```python
from build123d import *

# Parameters (mm, degrees)
F1_DEPTH = 190.5
F2_DEPTH = 127
F0_W     = 63.5
F0_H     = 63.5
F3_DEPTH = 101.6
F4_DEPTH = 25.4
F6_DEPTH = 63.5
F0_H_2   = 31.75
F7_DEPTH = 95.25


with BuildPart() as f1:
    # F0 (on Front) → F1 (new body)
    with BuildSketch(Plane.XZ):
        Polygon((0, 63.5), (0, 0), (95.25, 0), (95.25, 31.75), (158.75, 31.75), (158.75, 0), (254, 0), (254, 31.75), (317.5, 31.75), (317.5, 63.5), (254, 63.5), (190.5, 63.5), (127, 63.5), (63.5, 63.5), align=None)
    extrude(amount=F1_DEPTH)

    # F0 (on Front) → F2 (join)
    with BuildSketch(Plane.XZ):
        Polygon((0, 190.5), (0, 63.5), (63.5, 63.5), (63.5, 127), (63.5, 190.5), align=None)
    extrude(amount=F2_DEPTH)

    # F0 (on Front) → F3 (join)
    with BuildSketch(Plane.XZ):
        with Locations((95.25, 95.25)):
            Rectangle(F0_W, F0_H)
        with Locations((222.25, 95.25)):
            Rectangle(F0_W, F0_H)
    extrude(amount=F3_DEPTH)

    # F0 (on Front) → F4 (join)
    with BuildSketch(Plane.XZ):
        with Locations((158.75, 95.25)):
            Rectangle(F0_W, F0_H)
    extrude(amount=F4_DEPTH)

    # F5 (on face) → F6 (cut)
    with BuildSketch(Plane.XY.offset(127)):
        Polygon((254, -25.4), (190.5, -101.6), (254, -101.6), align=None)
    extrude(amount=-F6_DEPTH, mode=Mode.SUBTRACT)

    # F0 (on Front) → F7 (join)
    with BuildSketch(Plane.XZ):
        with Locations((285.75, 15.875)):
            Rectangle(F0_W, F0_H_2)
    extrude(amount=F7_DEPTH)


solid = f1.part
```
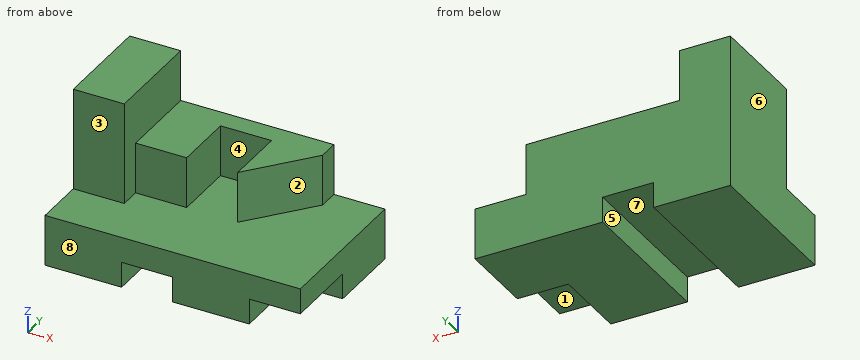
Geometry: final body of the model. Coordinates: model frame, mm. Face numbers are marked on the shaded views. A direction names the side the tool comes from. Round coordinates to 2 decimals unless told otherwise and drop trailing zeros. Loops run counter-clockwise (first coordinate to the right, second up) from the corner with the lowest first, then second, coordinate; pieces in that order, holes last.
Item 1: Section B-B, the plane y = -133.5. Output: boundary loops of the cut face in (x, z).
Checked values:
outline: (0, 0) - (95.25, 0) - (95.25, 31.75) - (158.75, 31.75) - (158.75, 0) - (254, 0) - (254, 31.75) - (317.5, 31.75) - (317.5, 63.5) - (0, 63.5) - close
Item 2: Mould query, pull axis X, two halves, no side actions, for the marked faces 6, 7 and 8. Classes: released by +X, released by -X, zero draft, split by the parting line, or undercut.
Checked values:
face 6: released by -X
face 7: undercut
face 8: zero draft
Item 3: Line query: L1, parallel to X at y = -102, z = 26.5; L2, parallel to Z at x = 255.5, y = -149.5; L3, parallel to Z at x = 282.5, y = -15. Output: solid intervals per line, ascending.
Checked values:
L1: x = 0 to 95.25, 158.75 to 254
L2: z = 31.75 to 63.5
L3: z = 0 to 63.5
Item 4: Section A-A, the plane z = 85. Output: boundary loops of the cut face in (x, y).
Checked values:
outline: (0, -127) - (63.5, -127) - (63.5, -101.6) - (127, -101.6) - (127, -25.4) - (190.5, -25.4) - (190.5, -101.6) - (254, -25.4) - (254, 0) - (0, 0) - close
Item 5: Contact query for flat-ended pins moving along their axis: P1, Ø20.5, axis at y = -13.5, z = 84.5, coming from the +X side; P2, Ø1.5, axis at y = -106, z = 131.5, coming from the -X side; P3, Ø19, axis at x = 173.5, z = 87, coming from the -Y side; P4, Ø16, axis at x = 280, z = 18, coming from the -Y side. Output: stop coordinate, or through.
Checked values:
P1: stops at x = 254
P2: stops at x = 0
P3: stops at y = -25.4
P4: stops at y = -95.25
Item 6: Reachability of the marked faces 1, 2, 3, 4 and 5 from +Z, -Z, +X, -X, +Y, -Y: full face, straight path, thin tool, end or side. Return the list, or none.
Checked values:
face 1: -Z, +X, -Y
face 2: +Z, +X, -Y
face 3: +Z, +X, -X, -Y
face 4: +Z, -Y
face 5: -Z, +Y, -Y
Item 7: Section D-D, the plane y = -87.5. Output: boundary loops of the cut face in (x, z).
Checked values:
outline: (0, 0) - (95.25, 0) - (95.25, 31.75) - (158.75, 31.75) - (158.75, 0) - (317.5, 0) - (317.5, 63.5) - (202.25, 63.5) - (202.25, 127) - (190.5, 127) - (190.5, 63.5) - (127, 63.5) - (127, 127) - (63.5, 127) - (63.5, 190.5) - (0, 190.5) - close
Item 8: Section C-C, the plane x = 263. Output: boundary loops of the cut face in (y, z).
Checked values:
outline: (-190.5, 31.75) - (-95.25, 31.75) - (-95.25, 0) - (0, 0) - (0, 63.5) - (-190.5, 63.5) - close
